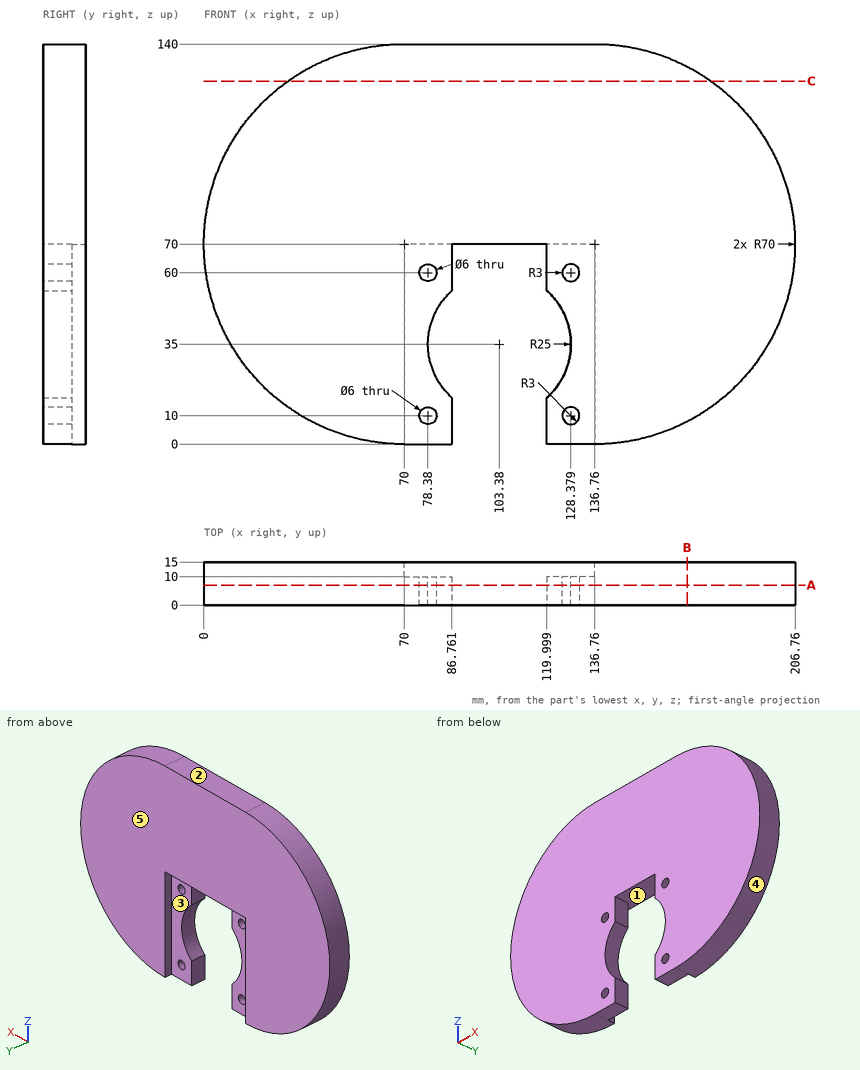
For this review, use the dimensioned drawing (mm, ordinates from the lowest corner) and the shaded views. A direction names the side the tool comes from. Coordinates: 2 decimals unless noted, no trailing zeros. Loops run counter-clockwise (first coordinate to the right, second up) from the corner with the lowest first, then second, coordinate; pieces in that order, holes last. Notation, with made-up numbers: (-11, 35) -> (2, 35) arc R10 ccw to (2, 54) -> close; hole circle Ø4 at (47.25, 64.5). An arc over 180 degrees is marked (long way). Return JSON: item names as keys, results as strings. Group by question number.
(1) For pin 1 Ø8 at (x, z) = (78.38, 60) entering from +Y; pin 2 Ø2 at (x, y) = (155, 9.5) entering from -Z; pin 3 Ø8 at (y, z) = (5, 64) entering from +X, all flat-tipped, find the tip position at first contact; note any pin that passes through.
(2) Consider section B-B, the plane x = 169. Give the boundary of the cut face in (y, z).
(3) Consider section A-A, the plane y = 7. Give the boundary of the cut face in (x, z) (1 decimal).
(4) Consider section C-C, the plane z = 127. Give the boundary of the cut face in (x, y).
(5) To check wall thickness, follow L1, parallel to Z at x = 129.5, y = 3.25; L2, parallel to Y at x = 133, z = 18.5; L3, parallel to Z at x = 109, y = 9. State the ranges of each line that lie inside material, in increasing order.
(6) Tool access review of the marked faces 1 and 2: name each direction out of +Z, -Z, +X, -X, +Y, -Y from which nothing blocks a thin tool from reaching the whole face with its end or side.
(7) Mouldability with a two-part tool opening along X and no side actions: class the marked faces 3, 4 and 5 as pulls with the +X half, pulls with the -X half, needs draft (parallel to the pull), parting line crosses it, or undercut.
Results below:
{
 "1": {"pin 1": "stops at y = 10", "pin 2": "stops at z = 2.16", "pin 3": "stops at x = 206.73"},
 "2": {"outline": "(0, 7.87) -> (15, 7.87) -> (15, 132.13) -> (0, 132.13) -> close"},
 "3": {"outline": "(70, 0) -> (86.8, 0) -> (86.8, 16.3) arc R25 cw to (86.8, 53.7) -> (86.8, 70) -> (120, 70) -> (120, 53.7) arc R25 cw to (120, 16.3) -> (120, 0) -> (136.8, 0) arc R70 ccw to (136.8, 140) -> (70, 140) arc R70 ccw to start; hole circle Ø6 at (78.4, 10); hole circle Ø6 at (78.4, 60); hole circle Ø6 at (128.4, 10); hole circle Ø6 at (128.4, 60)"},
 "4": {"outline": "(29.37, 0) -> (177.39, 0) -> (177.39, 15) -> (29.37, 15) -> close"},
 "5": {"L1": "z = 0 to 7.22, 12.78 to 57.22, 62.78 to 140", "L2": "y = 0 to 10", "L3": "z = 70 to 140"},
 "6": {"face 1": "-Z, +Y", "face 2": "+Z, +X, -X, +Y, -Y"},
 "7": {"face 3": "undercut", "face 4": "pulls with the +X half", "face 5": "needs draft"}
}
